Input: dimensioned drawing with shaded views. Units: mm. Origin: part minimum x, y, z. A direction names the side the tool comes from. Round coordinates to 2 decimals unless told otherwise and drop trailing zeros. Loops run counter-clockwise (first coordinate to the right, second up) from the corner with the lowest first, then second, coordinate; pieces in that order, holes last. Notation, with made-up numbers: (-25.5, 70) - (-15.5, 70) arc R12 ccw to (-15.5, 81) - close; hole circle Ø6 at (-24, 28). An arc over 180 degrees is marked (long way). One line per question, with ' | ' between items. Start each with the question number.
Item 1: Section A-A, the plane x = 60. Return loops of the section in (y, z) (3 decimals), plus the area to 3 significant figures.
Item 2: Material intervals for line 1 along Y through (x, z) = (60, 4.4) (3 decimals); line 2 along Y through (x, z) = (102, 4.2); line 3 along X through (y, z) = (57.5, 5.2) (3 decimals), sorted ascending.
Item 3: Set-up query: the marked faces 1 and 2. Return all of +Z, -Z, +X, -X, +Y, -Y with unobstructed straight access to the full face (end or side cutting, diameter ignored); none if empty.
Item 4: First-contact query: pin 1 (1 mm diameter, centred on y = 26.5, z = 3, fed in from +X); pin 2 (2.5 mm diameter, centred on x = 21.5, z = 4.5, fed in from +Y); pin 3 (1.5 mm diameter, centred on x = 28, z = 4, fed in from -Y). Flat tips, straight axial feed; report the tip coordinate or a pass-through.
Item 5: Draft query along X for the marked faces 3 and 4. Return one class per face: pulls with the +X half, pulls with the -X half, needs draft (parallel to the pull), parting line crosses it, or undercut.
Item 6: Section B-B, the plane y = 70. Return loops of the section in (x, z) (3 decimals), plus the area to 3 significant figures.
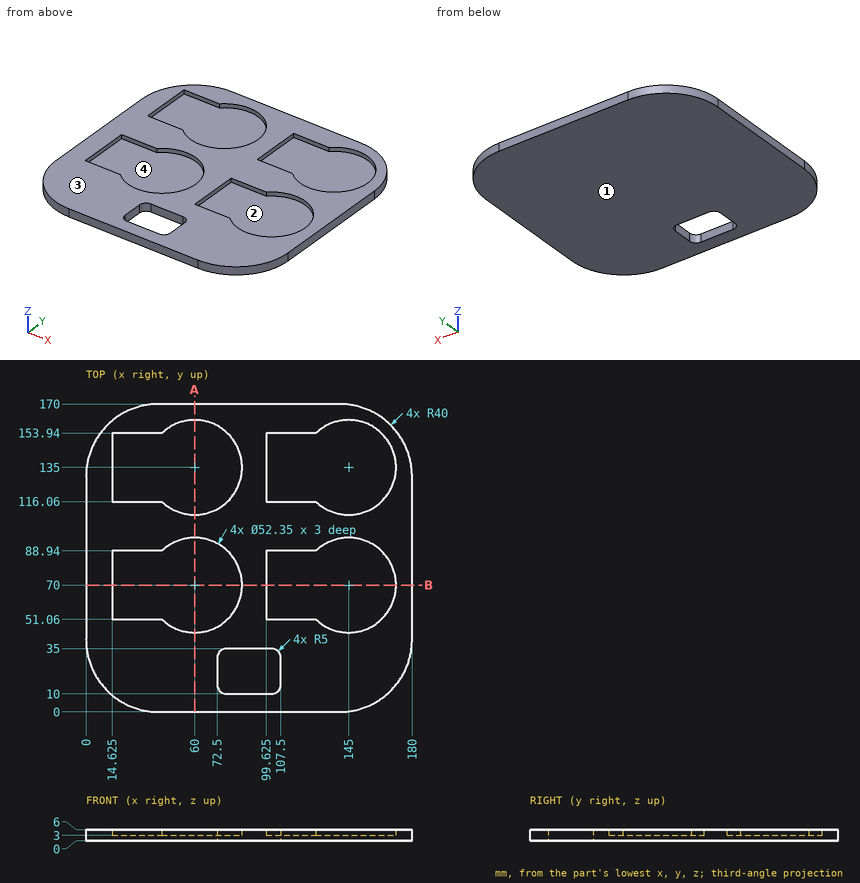
Return value:
1) outline: (0, 0) - (170, 0) - (170, 6) - (161.175, 6) - (161.175, 3) - (108.825, 3) - (108.825, 6) - (96.175, 6) - (96.175, 3) - (43.825, 3) - (43.825, 6) - (0, 6) - close | area: 706 mm2
2) line 1: 0 to 43.825, 96.175 to 108.825, 161.175 to 170 | line 2: 0 to 10, 35 to 51.06, 88.94 to 116.06, 153.94 to 170 | line 3: 0 to 14.625, 82.997 to 99.625, 167.997 to 180
3) face 1: -Z, +X, -X, +Y, -Y | face 2: +Z
4) pin 1: x = 177.83 | pin 2: y = 166.09 | pin 3: y = 1.61
5) face 3: needs draft | face 4: undercut
6) outline: (0, 0) - (180, 0) - (180, 6) - (171.175, 6) - (171.175, 3) - (99.625, 3) - (99.625, 6) - (86.175, 6) - (86.175, 3) - (14.625, 3) - (14.625, 6) - (0, 6) - close | area: 651 mm2
